```python
from build123d import *

# Parameters (mm, degrees)
SKETCH_W        = 62
SKETCH_H        = 34
PAD_DEPTH       = 40
SKETCH001_W     = 58
SKETCH001_H     = 30
POCKET_DEPTH    = 36
SKETCH002_W     = 45
SKETCH002_H     = 27
POCKET001_DEPTH = 5
POCKET002_DEPTH = 2
SKETCH004_R     = 1.5
POCKET003_DEPTH = 5
SKETCH005_W     = 5
SKETCH005_H     = 1
POCKET004_DEPTH = 5
SKETCH006_W     = 6
SKETCH006_H     = 2.5
PAD001_DEPTH    = 5
SKETCH007_W     = 6
SKETCH007_H     = 2.5
PAD002_DEPTH    = 5
SKETCH008_W     = 14
SKETCH008_H     = 8
POCKET005_DEPTH = 5
SKETCH009_W     = 35
SKETCH009_H     = 8
POCKET006_DEPTH = 5


with BuildPart() as part:
    # Sketch → Pad (new body)
    with BuildSketch(Plane.XY.offset(16)):
        with Locations((0, 12)):
            Rectangle(SKETCH_W, SKETCH_H)
    extrude(amount=PAD_DEPTH)

    # Sketch001 (on Face5 of Pad) → Pocket (cut)
    with BuildSketch(Plane(origin=(0, 0, 16), x_dir=(1, 0, 0), z_dir=(0, 0, -1))):
        with Locations((0, -12)):
            Rectangle(SKETCH001_W, SKETCH001_H)
    extrude(amount=-POCKET_DEPTH, mode=Mode.SUBTRACT)

    # Sketch002 (on Face5 of Pocket) → Pocket001 (cut)
    with BuildSketch(Plane.XY.offset(56)):
        with Locations((6.5, 11.5)):
            Rectangle(SKETCH002_W, SKETCH002_H)
    extrude(amount=-POCKET001_DEPTH, mode=Mode.SUBTRACT)

    # Sketch003 (on Face5 of Pocket001) → Pocket002 (cut)
    with BuildSketch(Plane.XY.offset(56)):
        Polygon((-16, 26), (29, 26), (29, -3), (-16, -3), (-16, 9), (-20, 9), (-20, 14), (-16, 14), align=None)
    extrude(amount=-POCKET002_DEPTH, mode=Mode.SUBTRACT)

    # Sketch004 (on Face29 of Pocket002) → Pocket003 (cut)
    with BuildSketch(Plane.XY.offset(54)):
        with Locations((-18, 11.5)):
            Circle(SKETCH004_R)
    extrude(amount=-POCKET003_DEPTH, mode=Mode.SUBTRACT)

    # Sketch005 (on Face14 of Pocket003) → Pocket004 (cut)
    with BuildSketch(Plane(origin=(29, 0, 0), x_dir=(0, -1, 0), z_dir=(-1, 0, 0))):
        with Locations((-19, 54.5)):
            Rectangle(SKETCH005_W, SKETCH005_H)
        with Locations((-5, 54.5)):
            Rectangle(SKETCH005_W, SKETCH005_H)
    extrude(amount=-POCKET004_DEPTH, mode=Mode.SUBTRACT)

    # Sketch006 (on Face18 of Pocket004) → Pad001 (join)
    with BuildSketch(Plane.XZ.offset(-27)):
        with Locations((-22, 31.25)):
            Rectangle(SKETCH006_W, SKETCH006_H)
        with Locations((22, 31.25)):
            Rectangle(SKETCH006_W, SKETCH006_H)
    extrude(amount=PAD001_DEPTH)

    # Sketch007 (on Face16 of Pad001) → Pad002 (join)
    with BuildSketch(Plane(origin=(0, -3, 0), x_dir=(-1, 0, 0), z_dir=(0, 1, 0))):
        with Locations((-22, 31.25)):
            Rectangle(SKETCH007_W, SKETCH007_H)
        with Locations((22, 31.25)):
            Rectangle(SKETCH007_W, SKETCH007_H)
    extrude(amount=PAD002_DEPTH)

    # Sketch008 (on Face2 of Pad002) → Pocket005 (cut)
    with BuildSketch(Plane(origin=(-31, 0, 0), x_dir=(0, -1, 0), z_dir=(-1, 0, 0))):
        with Locations((-7, 20)):
            Rectangle(SKETCH008_W, SKETCH008_H)
    extrude(amount=-POCKET005_DEPTH, mode=Mode.SUBTRACT)

    # Sketch009 (on Face9 of Pocket005) → Pocket006 (cut)
    with BuildSketch(Plane.XZ.offset(5)):
        with Locations((-0.5, 20)):
            Rectangle(SKETCH009_W, SKETCH009_H)
    extrude(amount=-POCKET006_DEPTH, mode=Mode.SUBTRACT)


with BuildPart() as part_1:
    # Body placement: moved
    add(part.part.moved(Location((0, 0, -36.5))))


solid = part_1.part
```
Can you work these out from the model? Positions are in its coordinate system, mm. A direction names the side the tool comes from. Round coordinates to 2 decimals unless told otherwise and drop trailing zeros. Loops run counter-clockwise (first coordinate to the right, second up) from the corner with the lowest first, then second, coordinate; pieces in that order, holes last.
Item 1: Suppose I cut it at A-A, the plane y = 11.5. Write out the boundary of the cut face in (x, z).
Item 2: Suppose I cut it at D-D, the plane z = -3. Write out the boundary of the cut face in (x, y).
Item 3: Suppose I cut it at C-C, the plane z = -14. Write out the boundary of the cut face in (x, y), then the cut area to 3 significant figures.
Item 4: Which directions (+Z, -Z, +X, -X, +Y, -Y) give clear straight access to the entire face, cutting with the end or side of a thin tool? Please do faces 5 (the flat face through (22, -1, -4)), 6 (the flat face through (17, -4, -17)), 7 (the flat face through (25, -1, -5)), 8 (the flat face through (-18, 13.2, 17.5)), 9 (the flat face through (-30, 7, -12.5)).
Item 5: Please list where these lines run through material, in increasing order: L1, parallel to Y at x = 5.5, z = -4.5; L2, parallel to X at y = 17.5, z = -15.5; L3, parallel to Y at x = -18, z = 16.
Item 6: Will these pins go through, and if not, where does the flat tip stop? pin 1 Ø5 at (x, y) = (-3, 22) entering from -Z; pin 2 Ø2 at (x, y) = (14, 25) entering from -Z; pin 3 Ø5.5 at (x, y) = (-20.5, 23.5) entering from -Z.
Item 7: If we mould it in two halves opening along Y, with no side actions, what happens to faces 1 (the flat face through (-18, 9, 19)), 2 (the flat face through (0, 29, -1)), 3 (the flat face through (22, 25, -6.5)), 4 (the flat face through (6.7, 27.2, -20.5))? For each: +Y half, -Y half, draft (parallel to the pull), parting line (faces both ways), or undercut.
Item 8: Suppose I cut it at B-B, the plane x = 14. Write out the boundary of the cut face in (y, z).
Reported:
1. outline: (-31, -12.5) - (-29, -12.5) - (-29, 15.5) - (-19.5, 15.5) - (-19.5, 17.5) - (-20, 17.5) - (-20, 19.5) - (-31, 19.5) - close; (-16.5, 15.5) - (-16, 15.5) - (-16, 17.5) - (-16.5, 17.5) - close; (29, -20.5) - (31, -20.5) - (31, 19.5) - (29, 19.5) - close
2. outline: (-31, -5) - (31, -5) - (31, 29) - (-31, 29) - close; hole (-29, -3) - (29, -3) - (29, 27) - (-29, 27) - close
3. outline: (-31, -5) - (-18, -5) - (-18, -3) - (-29, -3) - (-29, 0) - (-31, 0) - close; (-31, 14) - (-29, 14) - (-29, 27) - (29, 27) - (29, -3) - (17, -3) - (17, -5) - (31, -5) - (31, 29) - (-31, 29) - close
3. area: 270 mm2
4. face 5: none
4. face 6: -Z, -Y
4. face 7: -Z
4. face 8: +Z
4. face 9: -Z, -X
5. L1: y = -5 to -3, 27 to 29
5. L2: x = -31 to -29, 29 to 31
5. L3: y = -5 to 10, 13 to 29
6. pin 1: passes through
6. pin 2: stops at z = 15.5
6. pin 3: stops at z = -6.5
7. face 1: undercut
7. face 2: +Y half
7. face 3: undercut
7. face 4: draft
8. outline: (-5, -12.5) - (-3, -12.5) - (-3, 15.5) - (-2, 15.5) - (-2, 17.5) - (-3, 17.5) - (-3, 19.5) - (-5, 19.5) - close; (25, 15.5) - (27, 15.5) - (27, -20.5) - (29, -20.5) - (29, 19.5) - (26, 19.5) - (26, 17.5) - (25, 17.5) - close
